Here's how the part is built. I have some questions about the finished solid (model axes, mm). Round coordinates to 2 decimals unless told otherwise and drop trailing zeros. Write each loop counter-clockwise with the first axis right and the second up, starting at its lowest first coordinate (ties: lowest second). Pieces come first, ordered by that corner, then holes. Notation, with made-up numbers: M 30.5,32 L 64.5,32 A22 cw 64.5,68 Z; hole C -6,11 d10. An arc over 180 degrees is marked long. Use one line per item in the form item = value. Start each with the question number.
Q1. I'm going to push flat-ended pins straight in: pin 1 Ø1.6 at (x, y) = (126, 1) entering from -Z; pin 2 Ø1.6 at (y, z) = (1, -59.5) entering from +X; pin 3 Ø1.5 at (x, y) = (-106.5, 2.5) entering from +Z. Where does each tip first touch, or does it pass through?
Q2. I want a section at B-B on x = -17. List the corners of the cut face in (y, z) for me (3 decimals).
Q3. I want a section at D-D on x = 125. List the corners of the cut face in (y, z) for me (3 decimals).
Q4. I need wall thicknesses on line 1 along X through (y, z) = (0.7, 44); line 2 along X through (y, z) = (1.4, 97.5); line 3 along Z through (x, y) = (-0.5, 2.1). Which ranges of each line are inside material? Lowest first, please. Write a range as from..to.
Q5. I want a section at C-C on z = 33. List the corners of the cut face in (x, y) for me (3 decimals).
Q6. We'd pull the mould along X, two halves only. Please class faces 1 (the face through (62, 3.175, 22)), 2 (the face through (-73.495, 1.565, 125.197)), 3 (the face through (-72.18, 1.57, -77.99)): +X half, -X half, draft (parallel to the pull), parting line (faces both ways), or undercut.
Q7. I want a section at A-A on z = -46. List the corners of the cut face in (x, y) for me (3 decimals), and give its area (3 significant figures).
```python
from build123d import *

# Parameters (mm, degrees)
BOSS_EXTRUDE2_DEPTH = 3.175
SKETCH2_W           = 130.175
SKETCH2_H           = 5
CUT_EXTRUDE1_DEPTH  = 10


with BuildPart() as part:
    # Sketch1 → Boss-Extrude2 (new body)
    with BuildSketch(Plane(origin=(0, 0, 0), x_dir=(1, 0, 0), z_dir=(0, 1, 0))):
        with BuildLine():
            ThreePointArc((81.740740222, -99.802389706), (117.661764706, -125.202389706), (153.58278919, -99.802389706))
            Line((153.58278919, -99.802389706), (212.911764706, -99.802389706))
            Line((212.911764706, -99.802389706), (212.911764706, 52.597610294))
            Line((212.911764706, 52.597610294), (153.58278919, 52.597610294))
            ThreePointArc((153.58278919, 52.597610294), (117.661764706, 77.997610294), (81.740740222, 52.597610294))
            Line((81.740740222, 52.597610294), (-36.91721081, 52.597610294))
            ThreePointArc((-36.91721081, 52.597610294), (-72.838235294, 77.997610294), (-108.759259778, 52.597610294))
            Line((-108.759259778, 52.597610294), (-168.088235294, 52.597610294))
            Line((-168.088235294, 52.597610294), (-168.088235294, -23.602389706))
            Line((-168.088235294, -23.602389706), (-168.088235294, -99.802389706))
            Line((-168.088235294, -99.802389706), (-108.759259778, -99.802389706))
            ThreePointArc((-108.759259778, -99.802389706), (-72.838235294, -125.202389706), (-36.91721081, -99.802389706))
            Line((-36.91721081, -99.802389706), (81.740740222, -99.802389706))
        make_face()
        Polygon((-74.425735294, -87.102389706), (-71.250735294, -87.102389706), (-71.250735294, -98.214889706), (-60.138235294, -98.214889706), (-60.138235294, -101.389889706), (-71.250735294, -101.389889706), (-71.250735294, -112.502389706), (-74.425735294, -112.502389706), (-74.425735294, -101.389889706), (-85.538235294, -101.389889706), (-85.538235294, -98.214889706), (-74.425735294, -98.214889706), align=None, mode=Mode.SUBTRACT)
        Polygon((116.074264706, -87.102389706), (119.249264706, -87.102389706), (119.249264706, -98.214889706), (130.361764706, -98.214889706), (130.361764706, -101.389889706), (119.249264706, -101.389889706), (119.249264706, -112.502389706), (116.074264706, -112.502389706), (116.074264706, -101.389889706), (104.961764706, -101.389889706), (104.961764706, -98.214889706), (116.074264706, -98.214889706), align=None, mode=Mode.SUBTRACT)
        Polygon((-107.763235294, -43.446189706), (-107.763235294, -23.602389706), (-107.763235294, -3.758589706), (22.411764706, -3.758589706), (22.411764706, -43.446189706), align=None, mode=Mode.SUBTRACT)
        Polygon((-60.138235294, 54.185110294), (-60.138235294, 51.010110294), (-71.250735294, 51.010110294), (-71.250735294, 39.897610294), (-74.425735294, 39.897610294), (-74.425735294, 51.010110294), (-85.538235294, 51.010110294), (-85.538235294, 54.185110294), (-74.425735294, 54.185110294), (-74.425735294, 65.297610294), (-71.250735294, 65.297610294), (-71.250735294, 54.185110294), align=None, mode=Mode.SUBTRACT)
        Polygon((130.361764706, 54.185110294), (130.361764706, 51.010110294), (119.249264706, 51.010110294), (119.249264706, 39.897610294), (116.074264706, 39.897610294), (116.074264706, 51.010110294), (104.961764706, 51.010110294), (104.961764706, 54.185110294), (116.074264706, 54.185110294), (116.074264706, 65.297610294), (119.249264706, 65.297610294), (119.249264706, 54.185110294), align=None, mode=Mode.SUBTRACT)
    extrude(amount=BOSS_EXTRUDE2_DEPTH)

    # Sketch2 → Cut-Extrude1 (cut)
    with BuildSketch(Plane(origin=(0, 3.175, 0), x_dir=(1, 0, 0), z_dir=(0, 1, 0))):
        with Locations((-42.675735294, -45.946189706)):
            Rectangle(SKETCH2_W, SKETCH2_H)
        with Locations((-42.675735294, -1.258589706)):
            Rectangle(SKETCH2_W, SKETCH2_H)
    extrude(amount=-CUT_EXTRUDE1_DEPTH, mode=Mode.SUBTRACT)


solid = part.part
```
Reported:
q1.pin_1 = -77.24
q1.pin_2 = 150.8
q1.pin_3 = 106.3
q2.outline = M 0,-52.598 L 3.175,-52.598 L 3.175,-1.241 L 0,-1.241 Z; M 0,48.446 L 3.175,48.446 L 3.175,99.802 L 0,99.802 Z
q3.outline = M 0,-77.284 L 3.175,-77.284 L 3.175,-54.185 L 0,-54.185 Z; M 0,-51.01 L 3.175,-51.01 L 3.175,98.215 L 0,98.215 Z; M 0,101.39 L 3.175,101.39 L 3.175,124.489 L 0,124.489 Z
q4.line_1 = -168.09..-107.76, 22.41..212.91
q4.line_2 = -168.09..-74.43, -71.25..116.07, 119.25..212.91
q4.line_3 = -52.6..-1.24, 48.45..99.8
q5.outline = M -168.088,0 L -107.763,0 L -107.763,3.175 L -168.088,3.175 Z; M 22.412,0 L 212.912,0 L 212.912,3.175 L 22.412,3.175 Z
q6.face_1 = draft
q6.face_2 = undercut
q6.face_3 = undercut
q7.outline = M -168.088,0 L -74.426,0 L -74.426,3.175 L -168.088,3.175 Z; M -71.251,0 L 116.074,0 L 116.074,3.175 L -71.251,3.175 Z; M 119.249,0 L 212.912,0 L 212.912,3.175 L 119.249,3.175 Z
q7.area = 1,190 mm^2
